Input: part model. Units: mm. Frame: model coordinates. A direction names the side the tool comes from. Round coordinates to 2 decimals unless told otherwise and drop trailing zeros. Loops run counter-clockwise (first coordinate to the right, second up) from the corner with the lowest first, then second, coordinate; pieces in that order, holes last. Notation, with made-up numbers: M 73.5,-25.75 L 89.5,-25.75 A32 ccw 89.5,8.25 Z; hole C 53,-28.5 d5. An arc over 180 degrees is marked long. Use one line per item in the form item = value. Start each with the question number.
Q1. Section query D-D, the plane y = -20. Output: boundary loops of the cut face in (x, z), and give its area (4 significant figures).
Q2. Section query C-C, the plane z = 4.75. Output: boundary loops of the cut face in (x, y), and give its area (3 significant figures).
Q3. Section query B-B, the plane x = -12.5. Output: boundary loops of the cut face in (y, z).
Q4. Ray query, line 1 along Y through (x, z) = (-12.5, 1.8); line 2 along Y through (x, z) = (30.95, 11.5); line 3 along X through (y, z) = (44, 14). Return the intervals inside material, ascending.
Q5. Mould query, pull axis X, two halves, no side actions, for faces 4 (the cylindrical face through (53.75, -56.64, 1.52)), 5 (the flat face through (35.75, -0.8, 8.7)), 6 (the flat face through (3, 40, 10)), 7 (the flat face through (18, -50, 3)). Classes: pulls with the +X half, pulls with the -X half, needs draft (parallel to the pull), parting line crosses it, or undercut.
Q6. First-contact query: P1, Ø12, axis at x = -16, y = -53, coming from the +Z side; P2, Ø2.5, axis at y = 46.5, z = 11.5, coming from the +X side; P3, Ø8, axis at x = 28, y = 0, coming from the +Z side; P4, Ø2.5, axis at y = -11, z = 8.5, coming from the +X side. Flat tips, straight axial feed; report the tip coordinate or a pass-through.
Q7. Section query A-A, the plane y = 50. Output: boundary loops of the cut face in (x, z), and give its area (3 significant figures).
Q8. Access query for faces 1 (the flat face through (17, -42.5, 1)), 2 (the cylindrical face through (53.79, -43.4, 1.52)), 3 (the cylindrical face through (-2.95, 40.9, 13.84)). Directions: +Z, -Z, +X, -X, +Y, -Y. A direction counts if a zero-diameter tool reaches every point of the face in a straight line with its end or side. Return the directions, or none.
```python
from build123d import *

# Parameters (mm, degrees)
SKETCH_R          = 2
SKETCH_W          = 24.9
SKETCH_H          = 85
PAD_DEPTH         = 3
SKETCH001_W       = 4.15
SKETCH001_H       = 115
PAD001_DEPTH      = 11.7
SKETCH002_R       = 2
SKETCH002_W       = 80
SKETCH002_H       = 6
POCKET_DEPTH      = 50
POCKET_DEPTH_BACK = -100
SKETCH003_W       = 4
SKETCH003_H       = 115
PAD002_DEPTH      = 3.5
FILLET_R          = 3
FILLET001_R       = 3
FILLET002_R       = 3
FILLET003_R       = 3
FILLET004_R       = 3
FILLET005_R       = 3
FILLET006_R       = 3
FILLET007_R       = 3
FILLET008_R       = 3
FILLET009_R       = 3
FILLET010_R       = 3
FILLET011_R       = 3
FILLET012_R       = 3
FILLET013_R       = 3
FILLET014_R       = 3
FILLET015_R       = 3
FILLET016_R       = 3
FILLET017_R       = 3
FILLET018_R       = 3
FILLET019_R       = 3
FILLET020_R       = 3
FILLET021_R       = 3
FILLET022_R       = 3
FILLET023_R       = 3


with BuildPart() as part:
    # Sketch → Pad (new body)
    with BuildSketch(Plane.XY):
        Polygon((54.65, -57.5), (-20.35, -57.5), (-20.35, -42.5), (-5, -42.5), (-5, 42.5), (-20.35, 42.5), (-20.35, 57.5), (54.65, 57.5), (54.65, 42.5), (39.9, 42.5), (39.9, -42.5), (54.65, -42.5), align=None)
        with Locations((-12.5, 50)):
            Circle(SKETCH_R, mode=Mode.SUBTRACT)
        with Locations((47.5, 50)):
            Circle(SKETCH_R, mode=Mode.SUBTRACT)
        with Locations((-12.5, -50)):
            Circle(SKETCH_R, mode=Mode.SUBTRACT)
        with Locations((47.5, -50)):
            Circle(SKETCH_R, mode=Mode.SUBTRACT)
        with Locations((17.45, 0)):
            Rectangle(SKETCH_W, SKETCH_H, mode=Mode.SUBTRACT)
    extrude(amount=PAD_DEPTH)

    # Sketch001 → Pad001 (join)
    with BuildSketch(Plane.XY.offset(3)):
        with Locations((-2.925, 0)):
            Rectangle(SKETCH001_W, SKETCH001_H)
        with Locations((2.925, 0)):
            Rectangle(SKETCH001_W, SKETCH001_H)
        with Locations((31.975, 0)):
            Rectangle(SKETCH001_W, SKETCH001_H)
        with Locations((37.825, 0)):
            Rectangle(SKETCH001_W, SKETCH001_H)
    extrude(amount=PAD001_DEPTH)

    # Sketch002 → Pocket (cut, two sides)
    with BuildSketch(Plane.YZ.offset(5)) as pocket_sk:
        with Locations((-46.5, 11.5)):
            Circle(SKETCH002_R)
        with Locations((46.5, 11.5)):
            Circle(SKETCH002_R)
        with Locations((0, 12)):
            Rectangle(SKETCH002_W, SKETCH002_H)
    extrude(amount=-POCKET_DEPTH, mode=Mode.SUBTRACT)
    extrude(pocket_sk.sketch, amount=-POCKET_DEPTH_BACK, mode=Mode.SUBTRACT)

    # Sketch003 → Pad002 (join)
    with BuildSketch(Plane.XY.offset(3)):
        Rectangle(SKETCH003_W, SKETCH003_H)
        with Locations((35.05, 0)):
            Rectangle(SKETCH003_W, SKETCH003_H)
    extrude(amount=PAD002_DEPTH)

    # Fillet
    fillet_edges = [part.edges().sort_by_distance(p)[0] for p in [
        (-2.925, -57.5, 14.7),
    ]]
    fillet(fillet_edges, radius=FILLET_R)

    # Fillet001
    fillet001_edges = [part.edges().sort_by_distance(p)[0] for p in [
        (2.925, -57.5, 14.7),
    ]]
    fillet(fillet001_edges, radius=FILLET001_R)

    # Fillet002
    fillet002_edges = [part.edges().sort_by_distance(p)[0] for p in [
        (31.975, -57.5, 14.7),
    ]]
    fillet(fillet002_edges, radius=FILLET002_R)

    # Fillet003
    fillet003_edges = [part.edges().sort_by_distance(p)[0] for p in [
        (37.825, -57.5, 14.7),
    ]]
    fillet(fillet003_edges, radius=FILLET003_R)

    # Fillet004
    fillet004_edges = [part.edges().sort_by_distance(p)[0] for p in [
        (37.825, -40, 14.7),
    ]]
    fillet(fillet004_edges, radius=FILLET004_R)

    # Fillet005
    fillet005_edges = [part.edges().sort_by_distance(p)[0] for p in [
        (31.975, -40, 14.7),
    ]]
    fillet(fillet005_edges, radius=FILLET005_R)

    # Fillet006
    fillet006_edges = [part.edges().sort_by_distance(p)[0] for p in [
        (-2.925, -40, 14.7),
    ]]
    fillet(fillet006_edges, radius=FILLET006_R)

    # Fillet007
    fillet007_edges = [part.edges().sort_by_distance(p)[0] for p in [
        (2.925, -40, 14.7),
    ]]
    fillet(fillet007_edges, radius=FILLET007_R)

    # Fillet008
    fillet008_edges = [part.edges().sort_by_distance(p)[0] for p in [
        (54.65, -57.5, 1.5),
    ]]
    fillet(fillet008_edges, radius=FILLET008_R)

    # Fillet009
    fillet009_edges = [part.edges().sort_by_distance(p)[0] for p in [
        (54.65, -42.5, 1.5),
    ]]
    fillet(fillet009_edges, radius=FILLET009_R)

    # Fillet010
    fillet010_edges = [part.edges().sort_by_distance(p)[0] for p in [
        (54.65, 42.5, 1.5),
    ]]
    fillet(fillet010_edges, radius=FILLET010_R)

    # Fillet011
    fillet011_edges = [part.edges().sort_by_distance(p)[0] for p in [
        (54.65, 57.5, 1.5),
    ]]
    fillet(fillet011_edges, radius=FILLET011_R)

    # Fillet012
    fillet012_edges = [part.edges().sort_by_distance(p)[0] for p in [
        (37.825, 40, 14.7),
    ]]
    fillet(fillet012_edges, radius=FILLET012_R)

    # Fillet013
    fillet013_edges = [part.edges().sort_by_distance(p)[0] for p in [
        (31.975, 40, 14.7),
    ]]
    fillet(fillet013_edges, radius=FILLET013_R)

    # Fillet014
    fillet014_edges = [part.edges().sort_by_distance(p)[0] for p in [
        (37.825, 57.5, 14.7),
    ]]
    fillet(fillet014_edges, radius=FILLET014_R)

    # Fillet015
    fillet015_edges = [part.edges().sort_by_distance(p)[0] for p in [
        (31.975, 57.5, 14.7),
    ]]
    fillet(fillet015_edges, radius=FILLET015_R)

    # Fillet016
    fillet016_edges = [part.edges().sort_by_distance(p)[0] for p in [
        (2.925, 40, 14.7),
    ]]
    fillet(fillet016_edges, radius=FILLET016_R)

    # Fillet017
    fillet017_edges = [part.edges().sort_by_distance(p)[0] for p in [
        (-2.925, 40, 14.7),
    ]]
    fillet(fillet017_edges, radius=FILLET017_R)

    # Fillet018
    fillet018_edges = [part.edges().sort_by_distance(p)[0] for p in [
        (-2.925, 57.5, 14.7),
    ]]
    fillet(fillet018_edges, radius=FILLET018_R)

    # Fillet019
    fillet019_edges = [part.edges().sort_by_distance(p)[0] for p in [
        (2.925, 57.5, 14.7),
    ]]
    fillet(fillet019_edges, radius=FILLET019_R)

    # Fillet020
    fillet020_edges = [part.edges().sort_by_distance(p)[0] for p in [
        (-20.35, -57.5, 1.5),
    ]]
    fillet(fillet020_edges, radius=FILLET020_R)

    # Fillet021
    fillet021_edges = [part.edges().sort_by_distance(p)[0] for p in [
        (-20.35, -42.5, 1.5),
    ]]
    fillet(fillet021_edges, radius=FILLET021_R)

    # Fillet022
    fillet022_edges = [part.edges().sort_by_distance(p)[0] for p in [
        (-20.35, 42.5, 1.5),
    ]]
    fillet(fillet022_edges, radius=FILLET022_R)

    # Fillet023
    fillet023_edges = [part.edges().sort_by_distance(p)[0] for p in [
        (-20.35, 57.5, 1.5),
    ]]
    fillet(fillet023_edges, radius=FILLET023_R)


solid = part.part
```
Results found:
q1.outline = M -5,0 L 5,0 L 5,9 L 0.85,9 L 0.85,6.5 L -0.85,6.5 L -0.85,9 L -5,9 Z; M 29.9,0 L 39.9,0 L 39.9,9 L 35.75,9 L 35.75,6.5 L 34.05,6.5 L 34.05,9 L 29.9,9 Z
q1.area = 171.5 mm²
q2.outline = M -5,-57.5 L 5,-57.5 L 5,57.5 L -5,57.5 Z; M 29.9,-57.5 L 39.9,-57.5 L 39.9,57.5 L 29.9,57.5 Z
q2.area = 2,300 mm²
q3.outline = M -57.5,0 L -52,0 L -52,3 L -57.5,3 Z; M -48,0 L -42.5,0 L -42.5,3 L -48,3 Z; M 42.5,0 L 48,0 L 48,3 L 42.5,3 Z; M 52,0 L 57.5,0 L 57.5,3 L 52,3 Z
q4.line_1 = -57.5 to -52, -48 to -42.5, 42.5 to 48, 52 to 57.5
q4.line_2 = -57.5 to -48.5, -44.5 to -40, 40 to 44.5, 48.5 to 57.5
q4.line_3 = -5 to -0.85, 0.85 to 5, 29.9 to 34.05, 35.75 to 39.9
q5.face_4 = pulls with the +X half
q5.face_5 = undercut
q5.face_6 = needs draft
q5.face_7 = undercut
q6.P1 = 3
q6.P2 = through
q6.P3 = 9
q6.P4 = 39.9
q7.outline = M -20.35,0 L -14.5,0 L -14.5,3 L -20.35,3 Z; M -10.5,0 L 45.5,0 L 45.5,3 L 39.9,3 L 39.9,14.7 L 35.75,14.7 L 35.75,6.5 L 34.05,6.5 L 34.05,14.7 L 29.9,14.7 L 29.9,3 L 5,3 L 5,14.7 L 0.85,14.7 L 0.85,6.5 L -0.85,6.5 L -0.85,14.7 L -5,14.7 L -5,3 L -10.5,3 Z; M 49.5,0 L 54.65,0 L 54.65,3 L 49.5,3 Z
q7.area = 407 mm²
q8.face_1 = +Z, -Z
q8.face_2 = +Z, -Z, +X
q8.face_3 = +Z, +X, -X
